Part print with two shaded views. Sizes in mm from the minimum x, y, z corner. A direction names the side the tool comes from. Round coordinates to 2 decimals unless told otherwise and drop trailing zeros. Write each loop counter-clockwise with the first axis right and the second up, starting at its lowest first coordinate (ties: lowest second). Pieces come first, ordered by that corner, then holes. Notation, with made-up numbers: (44, 30.5) -> (102, 30.5) arc R8 ccw to (102, 38.5) -> close; hole circle Ø1 at (-37, 49.5). An arc over 180 degrees is marked (long way). Answer in a Markdown table with one row per item. Add a question column.
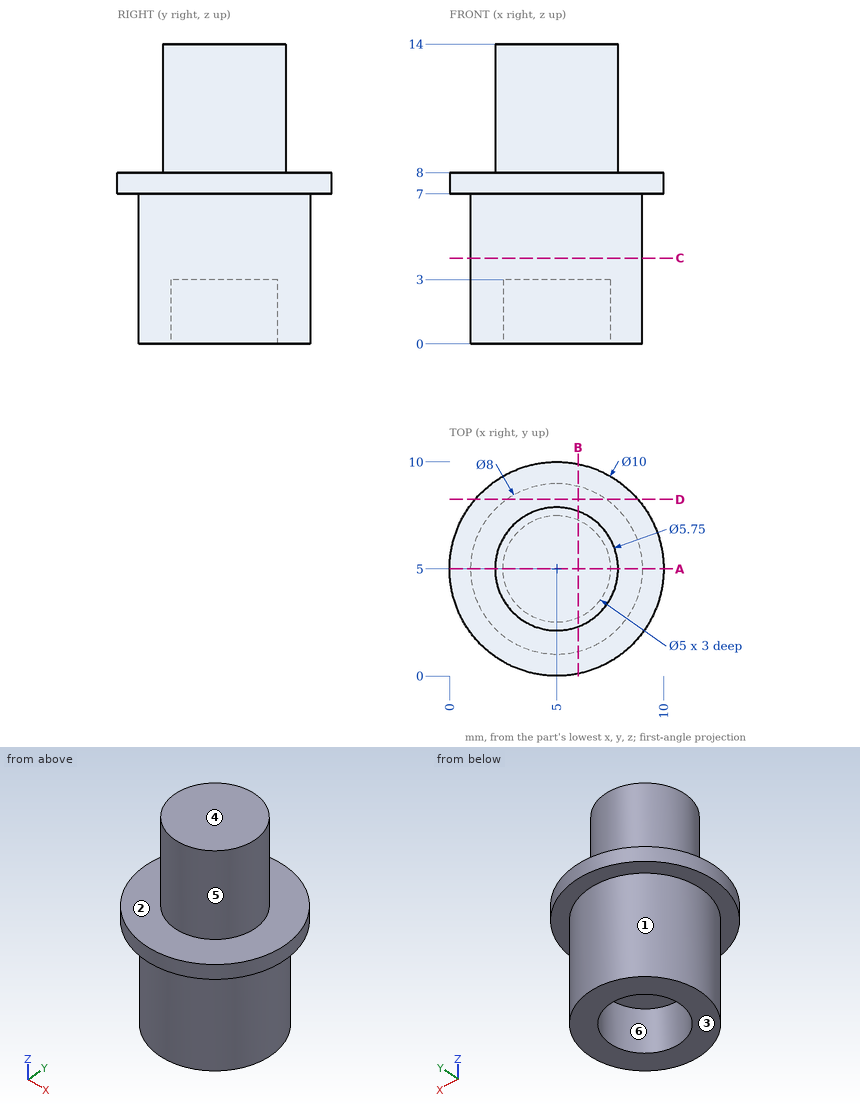
Item 1: Tool access for the marked faces 1, 2 and 3: list every direction of +Z, -Z, +X, -X, +Y, -Y with a clear straight run to the whole face (end or side of a thin tool).
Item 2: Pin check, flat tips, straight feed: pin 1 (5 mm diameter, centred on y = 5, z = 12, fed in from -X) (3 decimals); pin 2 (2 mm diameter, centred on y = 2, z = 4, fed in from +X); pin 3 (1 mm diameter, centred on y = 7, z = 4, fed in from +X). Stop position of each tip, or through.
Item 3: Saw through at A-A on y = 5. Give the cut face in (x, z) (3 decimals).
Item 4: Drill centre lines: probe 1 along X at (y, z) = (5, 2); probe 2 along Z at (x, y) = (2, 3); probe 3 along Y at (x, z) = (7, 1.75). Where is each one in solid material? Low to high.
Item 5: Saw through at D-D on y = 8.25. Give the cut face in (x, z), then the cut area to 3 significant figures.
Item 6: Saw through at B-B on x = 6. Give the cut face in (y, z).
Item 7: Saw through at C-C on z = 4. Give the cut face in (x, y).
Item 8: Two-plate mould, pull along X, no slides. Class the marked faces 4, 5 and 6: +X half, -X half, draft (parallel to the pull), parting line (faces both ways), or undercut.
Recorded:
| question | item | result |
|---|---|---|
| 1 | face 1 | -Z |
| 1 | face 2 | +Z |
| 1 | face 3 | -Z, +X, -X, +Y, -Y |
| 2 | pin 1 | x = 2.125 |
| 2 | pin 2 | x = 8.46 |
| 2 | pin 3 | x = 8.71 |
| 3 | outline | (0, 7) -> (1, 7) -> (1, 0) -> (2.5, 0) -> (2.5, 3) -> (7.5, 3) -> (7.5, 0) -> (9, 0) -> (9, 7) -> (10, 7) -> (10, 8) -> (7.875, 8) -> (7.875, 14) -> (2.125, 14) -> (2.125, 8) -> (0, 8) -> close |
| 4 | probe 1 | 1 to 2.5, 7.5 to 9 |
| 4 | probe 2 | 0 to 8 |
| 4 | probe 3 | 1.54 to 3.5, 6.5 to 8.46 |
| 5 | outline | (1.2, 7) -> (2.67, 7) -> (2.67, 0) -> (7.33, 0) -> (7.33, 7) -> (8.8, 7) -> (8.8, 8) -> (1.2, 8) -> close |
| 5 | area | 40.2 mm2 |
| 6 | outline | (0.1, 7) -> (1.13, 7) -> (1.13, 0) -> (2.71, 0) -> (2.71, 3) -> (7.29, 3) -> (7.29, 0) -> (8.87, 0) -> (8.87, 7) -> (9.9, 7) -> (9.9, 8) -> (7.7, 8) -> (7.7, 14) -> (2.3, 14) -> (2.3, 8) -> (0.1, 8) -> close |
| 7 | outline | circle Ø8 at (5, 5) |
| 8 | face 4 | draft |
| 8 | face 5 | parting line |
| 8 | face 6 | undercut |
